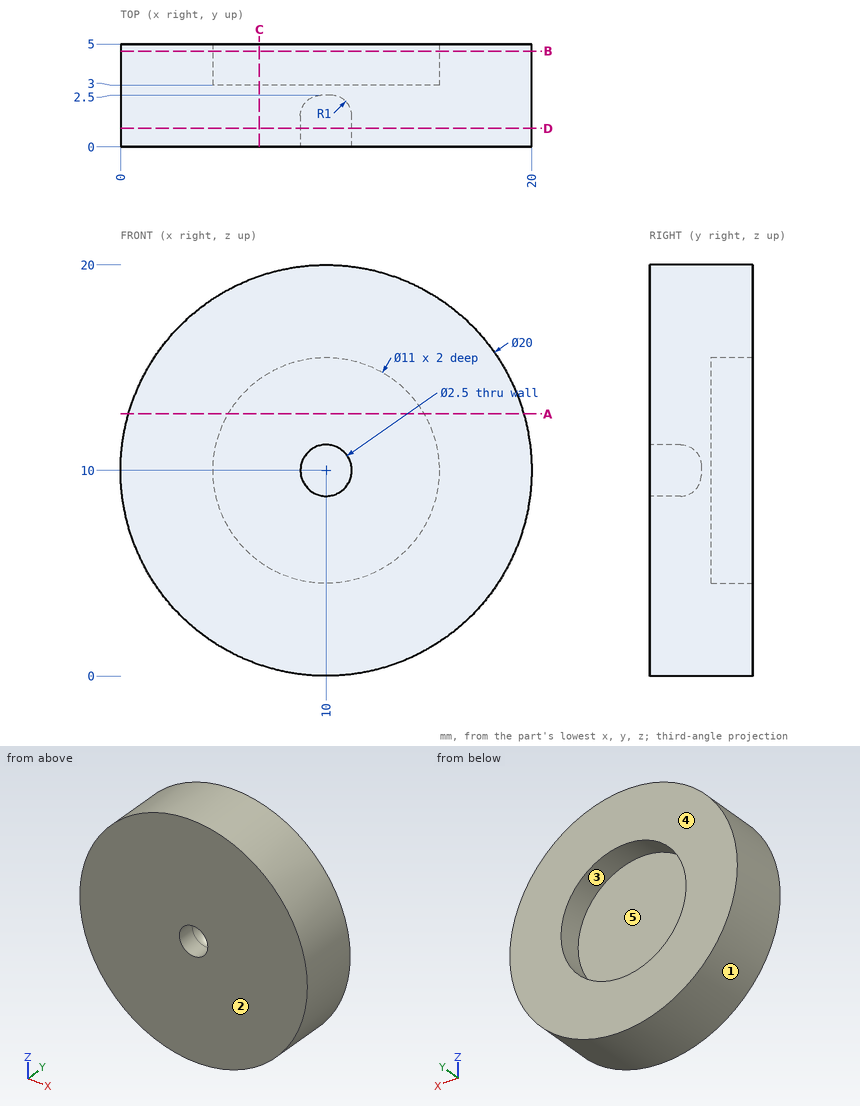
Geometry check sheet. Reference: drawing and pictorial views, mm from the part's lowest x, y, z. A direction names the side the tool comes from. Round coordinates to 2 decimals unless told otherwise and drop trailing zeros. Loops run counter-clockwise (first coordinate to the right, second up) from the corner with the lowest first, then second, coordinate; pieces in that order, holes last. Notation, with made-up numbers: (-26, 86.5) - (14, 86.5) arc R34 ccw to (14, 119.5) - close; hole circle Ø10 at (-30.5, 19.25). An arc over 180 degrees is marked (long way). Use a Markdown table: item, result.
Q1. Cross-section at A-A on z = 12.75. Record the cut outline in (x, y).
Solutions:
| item | result |
|---|---|
| outline | (0.39, 0) - (19.61, 0) - (19.61, 5) - (14.76, 5) - (14.76, 3) - (5.24, 3) - (5.24, 5) - (0.39, 5) - close |
Q2. Cross-section at C-C on x = 6.75. Record the cut outline in (y, z), plus the area to 3 significant figures.
Solutions:
| item | result |
|---|---|
| outline | (0, 0.54) - (5, 0.54) - (5, 5.56) - (3, 5.56) - (3, 14.44) - (5, 14.44) - (5, 19.46) - (0, 19.46) - close |
| area | 76.8 mm2 |
Q3. Cross-section at D-D on y = 0.9. Record the cut outline in (x, z).
Solutions:
| item | result |
|---|---|
| outline | circle Ø20 at (10, 10); hole circle Ø2.5 at (10, 10) |
Q4. Access from +Z, -Z, +X, -X, +Y, -Y to the whole of each face (thin tool, end or side, straight path). Record for the marked faces 4 and 5.
Solutions:
| item | result |
|---|---|
| face 4 | +Z, -Z, +X, -X, +Y |
| face 5 | +Y |
Q5. Draft check along Z on the marked faces 1, 2 and 3. Enter one of: released by +Z, released by -Z, zero draft, split by the parting line, or undercut.
Solutions:
| item | result |
|---|---|
| face 1 | split by the parting line |
| face 2 | zero draft |
| face 3 | undercut |
Q6. Material ranges on line 1 (X direction, y = 3.7, z = 10); line 2 (Y direction, x = 11, z = 7.75), recorded low to high.
Solutions:
| item | result |
|---|---|
| line 1 | x = 0 to 4.5, 15.5 to 20 |
| line 2 | y = 0 to 3 |
Q7. Cross-section at B-B on y = 4.65. Record the cut outline in (x, z), plus the area to 3 significant figures.
Solutions:
| item | result |
|---|---|
| outline | circle Ø20 at (10, 10); hole circle Ø11 at (10, 10) |
| area | 219 mm2 |
Q8. Go/stop test with flat-tipped pins: P1, Ø1.5, axis at x = 5, z = 17, coming from the -Y side; P2, Ø1, axis at y = 1.5, z = 18, coming from the -X side; P3, Ø3.5, axis at x = 12, z = 10, coming from the +Y side. Record where each tip stops, or that it passes through.
Solutions:
| item | result |
|---|---|
| P1 | stops at y = 0 |
| P2 | stops at x = 3.39 |
| P3 | stops at y = 3 |
